The listing builds one solid part. Answer for the finished solid, in the listing's coordinates (mm). A direction names the side the tool comes from. Round coordinates to 2 decimals unless told otherwise and drop trailing zeros. Write each loop counter-clockwise with the first axis right and the second up, starting at its lowest first coordinate (ties: lowest second). Pieces come first, ordered by that corner, then holes.
Autodesk Inventor part; units mm, degrees
ref_plane "YZ Plane" through (0, 0, 0) normal (1, 0, 0) x (0, 1, 0)
ref_plane "XZ Plane" through (0, 0, 0) normal (0, 1, 0) x (-1, 0, 0)
ref_plane "XY Plane" through (0, 0, 0) normal (0, 0, 1) x (1, 0, 0)
sketch "Skizze1" plane through (0, 0, 0) normal (0, 0, 1) x (1, 0, 0)
  circle A0 centre (0, 0) radius 35
  dimension "d0" = 70
extrude "Extrusion1" add sketch "Skizze1" along normal blind 100
sketch "Skizze2" plane through (0, 0, 100) normal (0, 0, 1) x (1, 0, 0)
  line L0 (10, -31) -> (12, -31)
  line L1 (12, -31) -> (12, 31)
  line L2 (12, 31) -> (10, 31)
  line L3 (10, 31) -> (10, -31)
  point P0 (0, 0)
  point P1 (10, 0)
  dimension "d3" = 2
  dimension "d4" = 62
  dimension "d5" = 10
extrude "Extrusion2" cut sketch "Skizze2" against normal blind 80
sketch "Skizze3" plane through (0, 0, 100) normal (0, 0, 1) x (1, 0, 0)
  line L0 (-15, -28.5) -> (18, -28.5)
  line L1 (18, -28.5) -> (18, 28.5)
  line L2 (18, 28.5) -> (-15, 28.5)
  line L3 (-15, 28.5) -> (-15, -28.5)
  line L4 (10, -31) -> (10, 31)
  point P0 (0, 0)
  point P1 (-15, 0)
  dimension "d8" = 8
  dimension "d9" = 57
  dimension "d10" = 25
extrude "Extrusion3" cut sketch "Skizze3" against normal blind 80
sketch "Skizze4" plane through (0, 0, 0) normal (0, 0, -1) x (-1, 0, 0)
  line L0 (-13.5, -13.5) -> (13.5, -13.5)
  line L1 (13.5, -13.5) -> (13.5, 13.5)
  line L2 (13.5, 13.5) -> (-13.5, 13.5)
  line L3 (-13.5, 13.5) -> (-13.5, -13.5)
  line L4 (-13.5, -13.5) -> (13.5, 13.5) construction
  line L5 (13.5, -13.5) -> (-13.5, 13.5) construction
  point P0 (0, 0)
  dimension "d13" = 27
  dimension "d14" = 27
extrude "Extrusion4" cut sketch "Skizze4" against normal blind 4
sketch "Skizze5" plane through (0, 0, 0) normal (0, 0, -1) x (-1, 0, 0)
  line L0 (-11, -11) -> (11, -11)
  line L1 (11, -11) -> (11, 11)
  line L2 (11, 11) -> (-11, 11)
  line L3 (-11, 11) -> (-11, -11)
  line L4 (-11, -11) -> (11, 11) construction
  line L5 (11, -11) -> (-11, 11) construction
  point P0 (0, 0)
  dimension "d17" = 22
  dimension "d18" = 22
extrude "Extrusion5" cut sketch "Skizze5" against normal blind 15
sketch "Skizze6" plane through (0, 0, 0) normal (0, 0, -1) x (-1, 0, 0)
  line L0 (14, 9) -> (8, 9)
  line L1 (8, 9) -> (8, -9)
  line L2 (8, -9) -> (14, -9)
  line L3 (14, -9) -> (14, 9)
  point P0 (0, 0)
  point P1 (8, 0)
  dimension "d22" = 8
  dimension "d23" = 6
  dimension "d24" = 18
extrude "Extrusion6" cut sketch "Skizze6" against normal through all
equation "\"d13\" = d14"
equation "\"d18\" = d17"
properties part number "Zack-Zack"
1. Section D-D on y = -16.5 is taken. Determine the outline of the cut face in (x, z).
Geometry says:
outline: (-30.87, 0) - (30.87, 0) - (30.87, 100) - (18, 100) - (18, 20) - (-15, 20) - (-15, 100) - (-30.87, 100) - close
2. Given pin 1 (2 mm diameter, centred on y = 12, z = 2, fed in from +X); pin 2 (1 mm diameter, centred on x = 11.5, z = 57.5, fed in from +Y); pin 3 (5 mm diameter, centred on y = 27, z = 72.5, fed in from +X) (3 decimals); pin 4 (1.5 mm diameter, centred on x = 28, y = -24, fed in from +Z), each flat-ended and moving along its own axis, determine where each tip first touches the part or whether it passes through.
Geometry says:
pin 1: stops at x = 33.23
pin 2: stops at y = 33.23
pin 3: stops at x = 24.995
pin 4: passes through
3. Section A-A on y = 0 is taken. Determine the outline of the cut face in (x, z), plus the area to 4 significant figures.
Geometry says:
outline: (-35, 0) - (-14, 0) - (-14, 20) - (-15, 20) - (-15, 100) - (-35, 100) - close; (-8, 15) - (11, 15) - (11, 4) - (13.5, 4) - (13.5, 0) - (35, 0) - (35, 100) - (18, 100) - (18, 20) - (-8, 20) - close
area: 3,945 mm2
4. Section C-C on z = 22.5 is taken. Determine the outline of the cut face in (x, y), plus the area to 3 significant figures.
Geometry says:
outline: circle Ø70 at (0, 0); hole (-15, -28.5) - (10, -28.5) - (10, -31) - (12, -31) - (12, -28.5) - (18, -28.5) - (18, 28.5) - (12, 28.5) - (12, 31) - (10, 31) - (10, 28.5) - (-15, 28.5) - close
area: 1,960 mm2
5. For a pull along Y with two mould halves and no side action, classify faces 4 (the face through (-14, 0, 10)), 5 (the face through (-28, 21, 49)), 6 (the face through (-16, 0, 100)) as released by +Y, released by -Y, zero draft, split by the parting line, or undercut.
Geometry says:
face 4: undercut
face 5: split by the parting line
face 6: zero draft
6. Straight lines are drawn through the part: line 1 along Z through (x, y) = (-7.5, 16.5); line 2 along X through (y, z) = (0.5, 96.5); line 3 along X through (y, z) = (-19.5, 94). For each, find the intervals that lie inside material, in ascending order.
Geometry says:
line 1: z = 0 to 20
line 2: x = -35 to -15, 18 to 35
line 3: x = -29.06 to -15, 18 to 29.06
7. A tool of negligible diameter and unlimited length cuts with its end or side. For faces 1 (the face through (0, -11, 9)), 2 (the face through (12, 30, 61)), 3 (the face through (-12, 9, 12)), from which of +Z, -Z, +X, -X, +Y, -Y can it reach the whole face along a straight path? Write none if from no direction.
Geometry says:
face 1: -Z
face 2: +Z
face 3: +Z, -Z
8. Section B-B on x = 0 is taken. Determine the outline of the cut face in (y, z), plus the area to 3 significant figures.
Geometry says:
outline: (-35, 0) - (-13.5, 0) - (-13.5, 4) - (-11, 4) - (-11, 15) - (11, 15) - (11, 4) - (13.5, 4) - (13.5, 0) - (35, 0) - (35, 100) - (28.5, 100) - (28.5, 20) - (-28.5, 20) - (-28.5, 100) - (-35, 100) - close
area: 2,090 mm2
